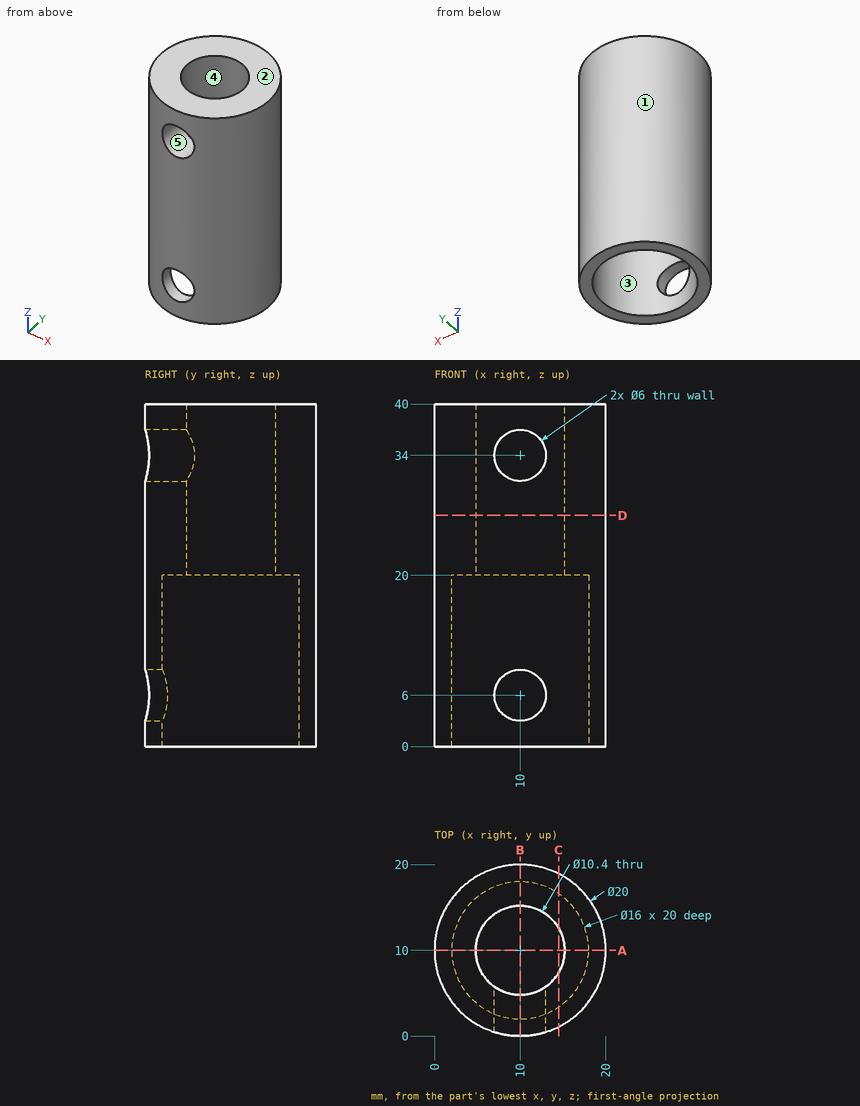
Print and shaded views of the part. All mm, measured from the part's lowest x, y and z. A direction names the side the tool comes from. Give positions to 0.01 mm unless a question says otherwise; leave off trailing zeros. Loops run counter-clockwise (first coordinate to the right, second up) from the corner with the lowest first, then second, coordinate; pieces in that order, holes last. Notation, with made-up numbers: M -2,-33.5 L 33,-33.5 A23 ccw 33,5.5 Z; hole C 73,3 d2. An arc over 180 degrees is marked long. Write each question's results on one line, items separated by ' | '.
Q1. Mould opens along X. For the marked faces 1, 2 and 3 say: pulls with the +X half, pulls with the -X half, needs draft (parallel to the pull), parting line crosses it, or undercut.
Geometry check:
face 1: parting line crosses it | face 2: needs draft | face 3: undercut
Q2. Which spindle directions (+Z, -Z, +X, -X, +Y, -Y) get a long thin tool onto all of the face, cutting with end or side? Do the marked faces 4 and 5. Say none if no direction does.
Geometry check:
face 4: +Z, -Z | face 5: -Y
Q3. Band-saw the part on D-D on z = 27. Write the cut outline in (x, y), and give its area (3 significant figures).
Geometry check:
outline: C 10,10 d20; hole C 10,10 d10.4 | area: 229 mm²
Q4. Band-saw the part on A-A on y = 10. Write the cut outline in (x, z).
Geometry check:
outline: M 0,0 L 2,0 L 2,20 L 4.8,20 L 4.8,40 L 0,40 Z; M 15.2,20 L 18,20 L 18,0 L 20,0 L 20,40 L 15.2,40 Z
Q5. Band-saw the part on C-C on x = 14.5. Write the cut outline in (y, z), and give its area (3 significant figures).
Geometry check:
outline: M 1.07,0 L 3.39,0 L 3.39,20 L 7.39,20 L 7.39,40 L 1.07,40 Z; M 12.61,20 L 16.61,20 L 16.61,0 L 18.93,0 L 18.93,40 L 12.61,40 Z | area: 346 mm²
Q6. Band-saw the part on B-B on x = 10. Write the cut outline in (y, z), and give its area (3 significant figures).
Geometry check:
outline: M 0,0 L 2,0 L 2,3 L 0,3 Z; M 0,9 L 2,9 L 2,20 L 4.8,20 L 4.8,31 L 0,31 Z; M 0,37 L 4.8,37 L 4.8,40 L 0,40 Z; M 15.2,20 L 18,20 L 18,0 L 20,0 L 20,40 L 15.2,40 Z | area: 231 mm²
Q7. Probe probe 1 along Y at (x, z) = (10, 29); probe 2 along X at (y, z) = (10.25, 2.5); probe 3 along X at (y, z) = (14.5, 5). List the from-to ranges inside material, lowest first.
Geometry check:
probe 1: y = 0 to 4.8, 15.2 to 20 | probe 2: x = 0 to 2, 18 to 20 | probe 3: x = 1.07 to 3.39, 16.61 to 18.93
Q8. Flat gauge pins, fed straight in: P1, Ø5, axis at x = 9, y = 6, coming from the -Z side; P2, Ø1, axis at x = 18, z = 34, coming from the +Y side; P3, Ø2, axis at x = 6.5, z = 20, coming from the -Y side. Where does each tip first touch, or does it go through?
Geometry check:
P1: stops at z = 20 | P2: stops at y = 16.61 | P3: stops at y = 0.32
